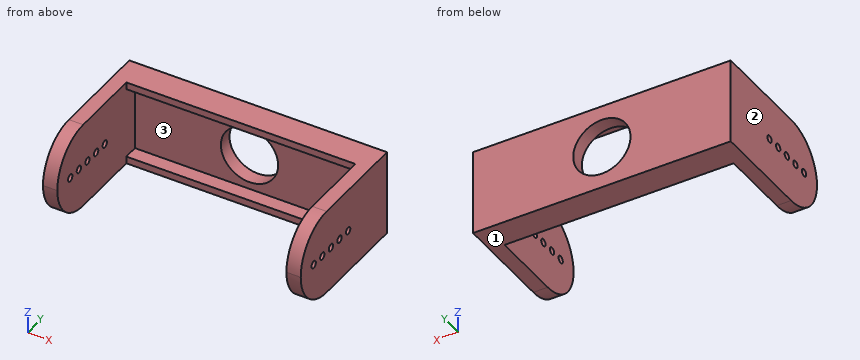
```python
from build123d import *

# Parameters (mm, degrees)
SKETCH1_W           = 36
SKETCH1_H           = 20
BOSS_EXTRUDE1_DEPTH = 12
SKETCH3_W           = 32
SKETCH3_H           = 16
CUT_EXTRUDE1_DEPTH  = 12
SKETCH4_W           = 32
SKETCH4_H           = 12
CUT_EXTRUDE2_DEPTH  = 12
CUT_EXTRUDE3_DEPTH  = 40.242833741
SKETCH5_R           = 4
CUT_EXTRUDE4_DEPTH  = 10
SKETCH6_R           = 0.5
CUT_EXTRUDE5_DEPTH  = 40.242833741
SKETCH7_W           = 32
SKETCH7_H           = 1
BOSS_EXTRUDE2_DEPTH = 2


with BuildPart() as part:
    # Sketch1 → Boss-Extrude1 (new body)
    with BuildSketch(Plane.XY):
        Rectangle(SKETCH1_W, SKETCH1_H)
    extrude(amount=BOSS_EXTRUDE1_DEPTH)

    # Sketch3 → Cut-Extrude1 (cut)
    with BuildSketch(Plane.XY.offset(12)):
        Rectangle(SKETCH3_W, SKETCH3_H)
    extrude(amount=-CUT_EXTRUDE1_DEPTH, mode=Mode.SUBTRACT)

    # Sketch4 → Cut-Extrude2 (cut)
    with BuildSketch(Plane(origin=(0, -8, 0), x_dir=(1, 0, 0), z_dir=(0, 1, 0))):
        with Locations((0, -6)):
            Rectangle(SKETCH4_W, SKETCH4_H)
    extrude(amount=-CUT_EXTRUDE2_DEPTH, mode=Mode.SUBTRACT)

    # Sketch2 → Cut-Extrude3 (cut, through all)
    with BuildSketch(Plane(origin=(18, 0, 0), x_dir=(0, 0, -1), z_dir=(1, 0, 0))):
        with BuildLine():
            Line((-12, -10), (-6, -10))
            ThreePointArc((-6, -10), (-10.242640687, -8.242640687), (-12, -4))
            Line((-12, -4), (-12, -10))
        make_face()
        with BuildLine():
            Line((-6, -10), (0, -10))
            Line((0, -10), (0, -4))
            ThreePointArc((0, -4), (-1.757359313, -8.242640687), (-6, -10))
        make_face()
    extrude(amount=-CUT_EXTRUDE3_DEPTH, mode=Mode.SUBTRACT)

    # Sketch5 → Cut-Extrude4 (cut)
    with BuildSketch(Plane(origin=(0, 10, 0), x_dir=(1, 0, 0), z_dir=(0, 1, 0))):
        with Locations(Location((0, -6, 0), (0, 0, 270))):
            Circle(SKETCH5_R)
    extrude(amount=-CUT_EXTRUDE4_DEPTH, mode=Mode.SUBTRACT)

    # Sketch6 → Cut-Extrude5 (cut, through all)
    with BuildSketch(Plane(origin=(18, 0, 0), x_dir=(0, 0, -1), z_dir=(1, 0, 0))):
        with Locations((-6, -7)):
            Circle(SKETCH6_R)
        with Locations((-6, -5)):
            Circle(SKETCH6_R)
        with Locations((-6, -3)):
            Circle(SKETCH6_R)
        with Locations((-6, -1)):
            Circle(SKETCH6_R)
        with Locations((-6, 1)):
            Circle(SKETCH6_R)
    extrude(amount=-CUT_EXTRUDE5_DEPTH, mode=Mode.SUBTRACT)

    # Sketch7 → Boss-Extrude2 (add)
    with BuildSketch(Plane.XZ.offset(-8)):
        with Locations((0, 11.5)):
            Rectangle(SKETCH7_W, SKETCH7_H)
        with Locations((0, 0.5)):
            Rectangle(SKETCH7_W, SKETCH7_H)
    extrude(amount=BOSS_EXTRUDE2_DEPTH)


solid = part.part
```
Read the model definition and answer for the solid it produces. Units are mm, in the model's axes. Face numbers are marked on the shaded views. Give positions to 0.01 mm unless a question says otherwise; leave off trailing zeros. Order: outer loops, then holes, each group sorted by start corner. A loop starts at its lowest first (then second) coordinate and runs counter-clockwise, first axis right, second up. Notation, with made-up numbers: (-4, 54.5) -> (51, 54.5) arc R16 ccw to (51, 72.5) -> close; hole circle Ø5 at (87, 52). An arc over 180 degrees is marked (long way). One line per item, written item: value. Start each with the question number.
(1) The part is cut by section B-B (y = -3). Determine the outline of the cut face in (x, z).
(2) Straight lines are drawn through the part: L1, parallel to Y at x = 17.1, z = 6; L2, parallel to X at y = -4, z = 4.5; L3, parallel to Y at x = 7.5, z = 2.25. For each, find the intervals that lie inside material, in ascending order.
(3) The part is cut by section A-A (x = 0). Determine the outline of the cut face in (y, z).
(4) For a pull along Z with two mould halves and no side action, classify the marked faces 1, 2 and 3 as released by +Z, released by -Z, zero draft, split by the parting line, or undercut.
(5) The part is cut by section D-D (z = 3.5). Determine the outline of the cut face in (x, y).
(6) Flat-ended cylindrical pins translate along their axes: P1, Ø0.5, axis at x = -2, z = 11.5, coming from the -Y side; P2, Ø5, axis at x = 0, z = 6, coming from the -Y side; P3, Ø3, axis at x = -1.5, z = 3.5, coming from the -Y side. Find the tip coordinate at first contact, or state that the pin passes through.
(7) The part is cut by section C-C (y = 4.75). Determine the outline of the cut face in (x, z).
Taken from the geometry:
1. outline: (-18, 0) -> (-16, 0) -> (-16, 5.5) -> (-18, 5.5) -> close; (-18, 6.5) -> (-16, 6.5) -> (-16, 12) -> (-18, 12) -> close; (16, 0) -> (18, 0) -> (18, 5.5) -> (16, 5.5) -> close; (16, 6.5) -> (18, 6.5) -> (18, 12) -> (16, 12) -> close
2. L1: -10 to -7.5, -6.5 to -5.5, -4.5 to -3.5, -2.5 to -1.5, -0.5 to 0.5, 1.5 to 10
2. L2: -18 to -16, 16 to 18
2. L3: 8 to 10
3. outline: (6, 0) -> (10, 0) -> (10, 2) -> (8, 2) -> (8, 1) -> (6, 1) -> close; (6, 11) -> (8, 11) -> (8, 10) -> (10, 10) -> (10, 12) -> (6, 12) -> close
4. face 1: released by -Z
4. face 2: zero draft
4. face 3: undercut
5. outline: (-18, -9.45) -> (-16, -9.45) -> (-16, 8) -> (-3.12, 8) -> (-3.12, 10) -> (-18, 10) -> close; (3.12, 8) -> (16, 8) -> (16, -9.45) -> (18, -9.45) -> (18, 10) -> (3.12, 10) -> close
6. P1: y = 6
6. P2: through
6. P3: y = 8
7. outline: (-18, 0) -> (-16, 0) -> (-16, 12) -> (-18, 12) -> close; (16, 0) -> (18, 0) -> (18, 12) -> (16, 12) -> close
